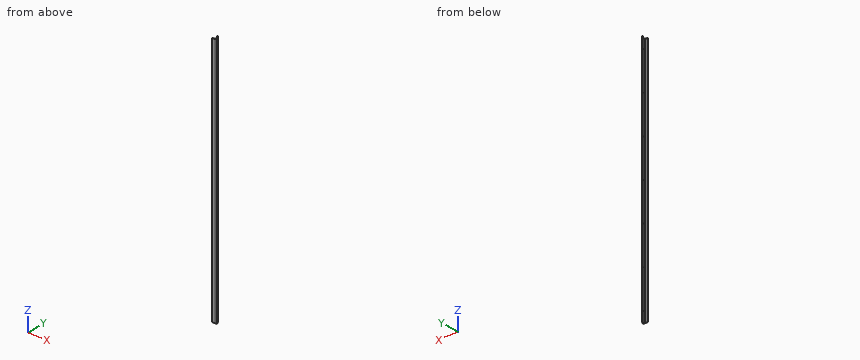
```python
from build123d import *

# Parameters (mm, degrees)
SM_BASE_FLANGE_1_DEPTH = 985
CUT_EXTRUDE_START      = 977
CUT_EXTRUDE_1_DEPTH    = 8
CUT_EXTRUDE_2_REACH    = 987.857
SKETCH_4_RX            = 3
SKETCH_4_RY            = 2.999814796


# Read off the part's stored shape, not the designer's step: Вырез-Вытянуть1
# Sheet-metal steps are written as plain solids
with BuildPart() as part:
    # Sketch 1 → Базовая кромка1 (new, symmetric)
    with BuildSketch(Plane.XY):
        with BuildLine():
            Line((-10.573213138, 28.075027408), (-4.074693371, 10.819523503))
            ThreePointArc((-4.074693371, 10.819523503), (-4.982758525, 3.447867974), (-11.561367346, 0))
            Line((-11.561367346, 0), (-30, 0))
            Line((-30, 0), (-30, 3))
            Line((-30, 3), (-11.561367346, 3))
            ThreePointArc((-11.561367346, 3), (-7.449736833, 5.154917483), (-6.882196111, 9.76220219))
            Line((-6.882196111, 9.76220219), (-13.380715879, 27.017706094))
            Line((-13.380715879, 27.017706094), (-10.573213138, 28.075027408))
        make_face()
    extrude(amount=SM_BASE_FLANGE_1_DEPTH, both=True)

    # Вырез-Вытянуть1 outline → Вырез-Вытянуть1 (cut)
    with BuildSketch(Plane.XY.offset(CUT_EXTRUDE_START)):
        with BuildLine():
            Line((-4.074693371, 10.819523503), (-6.882196111, 9.76220219))
            ThreePointArc((-6.882196111, 9.76220219), (-7.449736833, 5.154917483), (-11.561367346, 3))
            Line((-11.561367346, 3), (-30, 3))
            Line((-30, 3), (-30, 0))
            Line((-30, 0), (-11.561367346, 0))
            ThreePointArc((-11.561367346, 0), (-4.982758526, 3.447867973), (-4.074693371, 10.819523503))
        make_face()
    cut_extrude_1 = extrude(amount=CUT_EXTRUDE_1_DEPTH, mode=Mode.SUBTRACT)

    # Зеркальное отражение1: Вырез-Вытянуть1 across plane
    add(cut_extrude_1.mirror(Plane.XY), mode=Mode.SUBTRACT)

    # Эскиз4 → Вырез-Вытянуть2 (cut, up to next)
    with BuildSketch(Plane(origin=(0, 0, 0), x_dir=(0, 0, -1), z_dir=(0.9358342469192185, 0.3524404379368797, 0)), mode=Mode.PRIVATE) as cut_extrude_2_sk1:
        with Locations(Location((600, 20.076859002), (0, 0, 180))):
            Ellipse(SKETCH_4_RX, SKETCH_4_RY)
    cut_extrude_2_tool1 = extrude(cut_extrude_2_sk1.sketch, amount=-CUT_EXTRUDE_2_REACH, mode=Mode.PRIVATE) & part.part
    # Эскиз4 → Вырез-Вытянуть2 (cut, up to next)
    with BuildSketch(Plane(origin=(0, 0, 0), x_dir=(0, 0, -1), z_dir=(0.9358342469192185, 0.3524404379368797, 0)), mode=Mode.PRIVATE) as cut_extrude_2_sk2:
        with Locations(Location((300, 20.076859002), (0, 0, 180))):
            Ellipse(SKETCH_4_RX, SKETCH_4_RY)
    cut_extrude_2_tool2 = extrude(cut_extrude_2_sk2.sketch, amount=-CUT_EXTRUDE_2_REACH, mode=Mode.PRIVATE) & part.part
    # Эскиз4 → Вырез-Вытянуть2 (cut, up to next)
    with BuildSketch(Plane(origin=(0, 0, 0), x_dir=(0, 0, -1), z_dir=(0.9358342469192185, 0.3524404379368797, 0)), mode=Mode.PRIVATE) as cut_extrude_2_sk3:
        with Locations(Location((0, 20.076859002), (0, 0, 180))):
            Ellipse(SKETCH_4_RX, SKETCH_4_RY)
    cut_extrude_2_tool3 = extrude(cut_extrude_2_sk3.sketch, amount=-CUT_EXTRUDE_2_REACH, mode=Mode.PRIVATE) & part.part
    # Эскиз4 → Вырез-Вытянуть2 (cut, up to next)
    with BuildSketch(Plane(origin=(0, 0, 0), x_dir=(0, 0, -1), z_dir=(0.9358342469192185, 0.3524404379368797, 0)), mode=Mode.PRIVATE) as cut_extrude_2_sk4:
        with Locations((-300, 20.076859002)):
            Ellipse(SKETCH_4_RX, SKETCH_4_RY)
    cut_extrude_2_tool4 = extrude(cut_extrude_2_sk4.sketch, amount=-CUT_EXTRUDE_2_REACH, mode=Mode.PRIVATE) & part.part
    # Эскиз4 → Вырез-Вытянуть2 (cut, up to next)
    with BuildSketch(Plane(origin=(0, 0, 0), x_dir=(0, 0, -1), z_dir=(0.9358342469192185, 0.3524404379368797, 0)), mode=Mode.PRIVATE) as cut_extrude_2_sk5:
        with Locations((-600, 20.076859002)):
            Ellipse(SKETCH_4_RX, SKETCH_4_RY)
    cut_extrude_2_tool5 = extrude(cut_extrude_2_sk5.sketch, amount=-CUT_EXTRUDE_2_REACH, mode=Mode.PRIVATE) & part.part
    # Эскиз4 → Вырез-Вытянуть2 (cut, up to next)
    with BuildSketch(Plane(origin=(0, 0, 0), x_dir=(0, 0, -1), z_dir=(0.9358342469192185, 0.3524404379368797, 0)), mode=Mode.PRIVATE) as cut_extrude_2_sk6:
        with Locations((-900, 20.076859002)):
            Ellipse(SKETCH_4_RX, SKETCH_4_RY)
    cut_extrude_2_tool6 = extrude(cut_extrude_2_sk6.sketch, amount=-CUT_EXTRUDE_2_REACH, mode=Mode.PRIVATE) & part.part
    # Эскиз4 → Вырез-Вытянуть2 (cut, up to next)
    with BuildSketch(Plane(origin=(0, 0, 0), x_dir=(0, 0, -1), z_dir=(0.9358342469192185, 0.3524404379368797, 0)), mode=Mode.PRIVATE) as cut_extrude_2_sk7:
        with Locations(Location((900, 20.076859002), (0, 0, 180))):
            Ellipse(SKETCH_4_RX, SKETCH_4_RY)
    cut_extrude_2_tool7 = extrude(cut_extrude_2_sk7.sketch, amount=-CUT_EXTRUDE_2_REACH, mode=Mode.PRIVATE) & part.part
    add(cut_extrude_2_tool1.solids().sort_by_distance((-7.075897, 18.788612, -600))[0], mode=Mode.SUBTRACT)
    add(cut_extrude_2_tool2.solids().sort_by_distance((-7.075897, 18.788612, -300))[0], mode=Mode.SUBTRACT)
    add(cut_extrude_2_tool3.solids().sort_by_distance((-7.075897, 18.788612, 0))[0], mode=Mode.SUBTRACT)
    add(cut_extrude_2_tool4.solids().sort_by_distance((-7.075897, 18.788612, 300))[0], mode=Mode.SUBTRACT)
    add(cut_extrude_2_tool5.solids().sort_by_distance((-7.075897, 18.788612, 600))[0], mode=Mode.SUBTRACT)
    add(cut_extrude_2_tool6.solids().sort_by_distance((-7.075897, 18.788612, 900))[0], mode=Mode.SUBTRACT)
    add(cut_extrude_2_tool7.solids().sort_by_distance((-7.075897, 18.788612, -900))[0], mode=Mode.SUBTRACT)


solid = part.part
```
For this review, take the finished solid that the model builds, in its own axes (mm). Give positions to 0.01 mm unless a question says otherwise; leave off trailing zeros. Write each loop counter-clockwise with the first axis right and the second up, starting at its lowest first coordinate (ties: lowest second). Pieces come first, ordered by that corner, then holes.
Item 1: Wall thickness on probe 1 along X at (y, z) = (19, -260); probe 2 along X at (y, z) = (5.5, -657); probe 3 along Y at (x, z) = (-16, -331.5): over which ranges is each line inside the solid? List them lowest first.
Item 2: Take a section at B-B (x = -25.5). Give the boundary of the cut face in (y, z).
Item 3: Take a section at A-A (z = 854). Give the boundary of the cut face in (x, y), and give its area (3 significant figures).
Item 4: Insertion check: P1, Ø10, axis at x = -17.5, y = 4.5, coming from the +Z side; P2, Ø8.5, axis at x = -18, y = 4.5, coming from the -Z side; P3, Ø4, axis at y = 11.5, z = -104, coming from the -X side. Each pin has a flat end and moves straight along its axis. Give the tip position at first contact, or say it passes through.
Established:
1. probe 1: x = -10.36 to -7.16
1. probe 2: x = -7.23 to -3.96
1. probe 3: y = 0 to 3
2. outline: (0, -977) - (3, -977) - (3, 977) - (0, 977) - close
3. outline: (-30, 0) - (-11.56, 0) arc R8 ccw to (-4.07, 10.82) - (-10.57, 28.08) - (-13.38, 27.02) - (-6.88, 9.76) arc R5 cw to (-11.56, 3) - (-30, 3) - close
3. area: 148 mm2
4. P1: stops at z = 977
4. P2: stops at z = -977
4. P3: stops at x = -8.29
